Autodesk Fusion 360 part; units mm, degrees
sketch "Sketch1" plane through (0, 0, 0) normal (0, 0, 1) x (1, 0, 0)
  line L0 (0, 0) -> (25.5, 0)
  line L1 (25.5, 0) -> (25.5, -10.6)
  line L2 (25.5, -10.6) -> (0, -10.6)
  line L3 (0, -10.6) -> (0, 0)
  dimension "d1" = 10.6
  dimension "d2" = 25.5
extrude "Extrude1" add sketch "Sketch1" along normal blind 1
sketch "Sketch2" plane through (0, 0, 1) normal (0, 0, 1) x (-1, 0, 0)
  line L0 (0, 10.6) -> (-25.5, 10.6)
  line L1 (-25.5, 10.6) -> (-25.5, 0)
  line L2 (-25.5, 0) -> (0, 0)
  line L3 (0, 0) -> (0, 10.6)
  line L4 (-0.5, 0.5) -> (-25, 0.5)
  line L5 (-25, 0.5) -> (-25, 10.1)
  line L6 (-25, 10.1) -> (-0.5, 10.1)
  line L7 (-0.5, 10.1) -> (-0.5, 0.5)
  line L8 (-25.5, 10.6) -> (0, 10.6)
  dimension "d5" = 0.5
  dimension "d6" = 0.5
  dimension "d26" = 0.5
  dimension "d27" = 0.5
extrude "Extrude2" add sketch "Sketch2" along normal blind 25
sketch "Sketch3" plane through (0, 0, 0) normal (0, 0, -1) x (1, 0, 0)
  line L0 (25.5, 10.6) -> (0, 10.6)
  line L1 (0, 10.6) -> (0, 0)
  line L2 (0, 0) -> (25.5, 0)
  line L3 (25.5, 0) -> (25.5, 10.6)
  line L4 (7.25, 8.3) -> (18.25, 8.3)
  line L5 (18.25, 8.3) -> (18.25, 2.3)
  line L6 (18.25, 2.3) -> (7.25, 2.3)
  line L7 (7.25, 2.3) -> (7.25, 8.3)
  dimension "d12" = 11
  dimension "d13" = 6
  dimension "d14" = 2.3
  dimension "d15" = 7.25
  dimension "d28" = 25.5
  dimension "d29" = 10.6
extrude "Extrude3" cut sketch "Sketch3" against normal blind 11 contours L4 L5 L6 L7
fillet "Fillet1" radius 1.8 4 edges at (25, -10.1, 13.5) (0.5, -0.5, 13.5) (0.5, -10.1, 13.5) (25, -0.5, 13.5)
fillet "Fillet2" radius 1.8 4 edges at (0, -10.6, 13) (25.5, -10.6, 13) (25.5, 0, 13) (0, 0, 13)
fillet "Fillet3" radius 0.7 8 edges at (0.5272, -10.0728, 0) (0, -5.3, 0) (0.5272, -0.5272, 0) (12.75, 0, 0) (24.9728, -0.5272, 0) (25.5, -5.3, 0) (24.9728, -10.0728, 0) (12.75, -10.6, 0)
equation "d14 = ( d29 - d13 ) / 2"
equation "d15 = ( d28 - d12 ) / 2"
Work out the finished part from the listing and answer in its coordinate system (mm). A direction names the side the tool comes from. Coordinates: 2 decimals unless noted, no trailing zeros. Write each loop counter-clockwise with the first axis right and the second up, starting at its lowest first coordinate (ties: lowest second). Pieces come first, ordered by that corner, then holes. Notation, with made-up numbers: (56.5, -5) - (69.5, -5) arc R21 cw to (69.5, 28) - close; hole circle Ø4 at (-29.5, -30). An arc over 180 degrees is marked (long way). Answer as a JSON object with one key per item and string values.
Q1. Which of the six approach directions +Z, -Z, +X, -X, +Y, -Y give full straight-line access (tool end or side, diameter ignored) to faces 4 (the cylindrical face through (24.487, -1.041, 13.675)), 5 (the flat face through (7.25, -5.3, 0.5)), 6 (the cylindrical face through (24.987, -10.059, 13.173))?
Results list:
{"face 4": "+Z", "face 5": "+Z, -Z", "face 6": "+Z, -Z, +X, -Y"}
Q2. Find section C-C (z = 13). Write down the section's boundary in (x, y), plus the area to 3 significant figures.
Results list:
{"outline": "(0, -8.8) arc R1.8 ccw to (1.8, -10.6) - (23.7, -10.6) arc R1.8 ccw to (25.5, -8.8) - (25.5, -1.8) arc R1.8 ccw to (23.7, 0) - (1.8, 0) arc R1.8 ccw to (0, -1.8) - close; hole (0.5, -8.3) arc R1.8 ccw to (2.3, -10.1) - (23.2, -10.1) arc R1.8 ccw to (25, -8.3) - (25, -2.3) arc R1.8 ccw to (23.2, -0.5) - (2.3, -0.5) arc R1.8 ccw to (0.5, -2.3) - close", "area": "35.1 mm^2"}
Q3. Find section A-A (x = 8). Write down the section's boundary in (y, z).
Results list:
{"outline": "(-10.6, 0.7) arc R0.7 ccw to (-9.9, 0) - (-8.3, 0) - (-8.3, 1) - (-10.1, 1) - (-10.1, 26) - (-10.6, 26) - close; (-2.3, 0) - (-0.7, 0) arc R0.7 ccw to (0, 0.7) - (0, 26) - (-0.5, 26) - (-0.5, 1) - (-2.3, 1) - close"}
Q4. Given pin 1 Ø2 at (x, z) = (15, 11.5) entering from +Y; pin 2 Ø3 at (x, y) = (12, -7.5) entering from +Z, each flat-ended and moving along its own axis, determine where each tip first touches the part or whether it passes through.
Results list:
{"pin 1": "stops at y = 0", "pin 2": "stops at z = 1"}
Q5. For a pull along X with two mould halves and no side action, classify faces 1 (the cylindrical face through (1.041, -1.013, 13.675)), 2 (the cylindrical face through (0.513, -10.059, 13.527)), 3 (the flat face through (14.7, -10.4, 26)) as pulls with the +X half, pulls with the -X half, needs draft (parallel to the pull), parting line crosses it, or undercut.
Results list:
{"face 1": "undercut", "face 2": "pulls with the -X half", "face 3": "needs draft"}
Q6. Find section B-B (y = -5.25). Write down the section's boundary in (x, z).
Results list:
{"outline": "(0, 0.7) arc R0.7 ccw to (0.7, 0) - (7.25, 0) - (7.25, 1) - (0.5, 1) - (0.5, 26) - (0, 26) - close; (18.25, 0) - (24.8, 0) arc R0.7 ccw to (25.5, 0.7) - (25.5, 26) - (25, 26) - (25, 1) - (18.25, 1) - close"}
Q7. Consider L1, parallel to Y at x = 7.75, z = 1.5; L2, parallel to X at y = -7, z = 9; L3, parallel to Z at x = 2.5, y = -6.75. Determine where each line is inside the solid, lowest interval first. Write a range as from..to.
Results list:
{"L1": "y = -10.6..-10.1, -0.5..0", "L2": "x = 0..0.5, 25..25.5", "L3": "z = 0..1"}
Q8. Find section D-D (x = 3.5). Write down the section's boundary in (y, z).
Results list:
{"outline": "(-10.6, 0.7) arc R0.7 ccw to (-9.9, 0) - (-0.7, 0) arc R0.7 ccw to (0, 0.7) - (0, 26) - (-0.5, 26) - (-0.5, 1) - (-10.1, 1) - (-10.1, 26) - (-10.6, 26) - close"}
